Input: part model. Units: mm. Frame: model coordinates. A direction names the side the tool comes from. Round coordinates to 2 decimals unless told otherwise and drop trailing zeros. Loops run counter-clockwise (first coordinate to the right, second up) from the corner with the lowest first, then second, coordinate; pieces in that order, holes last. Notation, with made-up numbers: (-25.75, 66) -> (3.25, 66) arc R22 cw to (3.25, 94) -> close; hole circle Ø6 at (-9.5, 81.5). An arc over 180 degrees is marked (long way). One line per question, with ' | ' between items. Start each with the question number.
Q1. Material intervals for L1, parallel to X at y = 36, z = 0; L2, parallel to Z at x = 0, y = 36; L3, parallel to Y at x = 17.5, z = 17, sorted ascending.
Q2. Cut plane A-A on z = 0. Return loops of the section in (x, y).
Q3. Cut plane B-B on y = 28.5. Return loops of the section in (x, z).
Q4. Cut plane C-C on y = 14. Return loops of the section in (x, z), and give its area (3 significant figures).
Q5. Contact query for flat-ended pins moving along their axis: P1, Ø12, axis at y = 23, z = -3, coming from the +X side; P2, Ø23, axis at x = 0, z = 0, coming from the -Y side; P3, Ø10, axis at x = 15, y = 24, coming from the +Z side; P4, Ø8, axis at x = -14, z = 2.5, coming from the +Y side. Output: stop coordinate, or through.
Q6. Access query for faces 1 (the face through (10, 35, -8)), 2 (the face through (-9.76, 35.99, -2.17)). Directions: +Z, -Z, +X, -X, +Y, -Y. A direction counts if a zero-diameter tool reaches every point of the face in a straight line with its end or side. Return the directions, or none.
Q7. Mould query, pull axis X, two halves, no side actions, for faces 3 (the face through (17, 18, -37)), 4 (the face through (-8.696, 37.313, 5.544)), 5 (the face through (38.738, 38.042, 9.967)), 6 (the face through (-45.84, 2.54, -1.01)). Classes: pulls with the +X half, pulls with the -X half, needs draft (parallel to the pull), parting line crosses it, or undercut.
from build123d import *
from OCP.BRepFilletAPI import BRepFilletAPI_MakeChamfer

# Parameters (mm, degrees)
REVOLVE1_ANGLE          = 180
BOSS_EXTRUDE1_DEPTH     = 60
CUT_EXTRUDE2_DEPTH      = 87.407305825
CUT_EXTRUDE2_DEPTH_BACK = 87.407305825
SKETCH8_R               = 10
BOSS_EXTRUDE2_DEPTH     = 7
CHAMFER1_SIZE           = 5
CHAMFER1_SIZE2          = 6.012778745
CHAMFER2_SIZE           = 1
CHAMFER2_SIZE2          = 0.800998829
CHAMFER2_SIZE2_2        = 1.505173624
CHAMFER2_SIZE2_3        = 0.802603699
CHAMFER2_SIZE2_4        = 1.49466769


with BuildPart() as part:
    # Sketch2 → Revolve1 (revolve)
    with BuildSketch(Plane(origin=(0, 0, 0), x_dir=(0, 0, -1), z_dir=(1, 0, 0))):
        Polygon((37, 0), (45.85, 0), (45.85, 5), (40, 42), (0, 42), (0, 35), (37, 35), align=None)
    revolve(axis=Axis((0, 0, 0), (0, 1, 0)), revolution_arc=REVOLVE1_ANGLE)

    # Sketch7 → Boss-Extrude1 (add)
    with BuildSketch(Plane(origin=(0, 0, 0), x_dir=(0, 0, -1), z_dir=(1, 0, 0))):
        Polygon((-37, 0), (-37, 35), (37, 35), (37, 0), (45.85, 0), (45.85, 5), (40, 42), (-40, 42), (-45.85, 5), (-45.85, 0), align=None)
    extrude(amount=BOSS_EXTRUDE1_DEPTH)

    # Sketch8 → Cut-Extrude2 (cut, two sides: drawn at the far end of the back side and taken through both)
    with BuildSketch(Plane(origin=(0, 0, 0), x_dir=(1, 0, 0), z_dir=(0, 1, 0)).offset(-CUT_EXTRUDE2_DEPTH_BACK)):
        with Locations(Location((0, 0, 0), (0, 0, 270))):
            Circle(SKETCH8_R)
        Polygon((10, -45.85), (38, 45.85), (138, 45.85), (138, -45.85), align=None)
    extrude(amount=CUT_EXTRUDE2_DEPTH + CUT_EXTRUDE2_DEPTH_BACK, mode=Mode.SUBTRACT)

    # Sketch9 → Boss-Extrude2 (add)
    with BuildSketch(Plane(origin=(0, 42, 0), x_dir=(1, 0, 0), z_dir=(0, 1, 0))):
        with BuildLine():
            Line((31.519782555, 24.627287867), (0, -40))
            ThreePointArc((0, -40), (35.951992397, -17.534373175), (31.519782555, 24.627287867))
        make_face()
    extrude(amount=-BOSS_EXTRUDE2_DEPTH)

    # Chamfer1: one chamfer whose edges measure the first distance from different faces: ONE call of the kernel's chamfer builder (chamfer() names one face for all edges)
    chamfer1_edges_1 = [part.edges().sort_by_distance(p)[0] for p in [
        (-40, 42, 0),
        (5.893129771, 42, 40),
        (18.106870229, 42, -40),
    ]]
    chamfer1_side_1 = [part.faces().sort_by_distance(p)[0] for p in [
        (18.106870229, 42, -38.86862915),
    ]]
    chamfer1_edges_2 = [part.edges().sort_by_distance(p)[0] for p in [
        (0, 42, -10),
        (33.866761506, 42, -32.313643934),
    ]]
    chamfer1 = BRepFilletAPI_MakeChamfer(part.part.solid().wrapped)
    for e in chamfer1_edges_1:
        chamfer1.Add(CHAMFER1_SIZE, CHAMFER1_SIZE2, e.wrapped, chamfer1_side_1[0].wrapped)  # the first distance lies on this face
    for e in chamfer1_edges_2:
        chamfer1.Add(CHAMFER1_SIZE, e.wrapped)
    add(Compound.cast(chamfer1.Shape()), mode=Mode.REPLACE)

    # Chamfer2: one chamfer whose edges measure the first distance from different faces: ONE call of the kernel's chamfer builder (chamfer() names one face for all edges)
    chamfer2_edges_1 = [part.edges().sort_by_distance(p)[0] for p in [
        (39.67158228, 42, 5.115228187),
    ]]
    chamfer2_edges_2 = [part.edges().sort_by_distance(p)[0] for p in [
        (12.702290076, 17.5, 37),
    ]]
    chamfer2_side_2 = [part.faces().sort_by_distance(p)[0] for p in [
        (11.622460622, 15.898187568, 40.536441463),
    ]]
    chamfer2_edges_3 = [part.edges().sort_by_distance(p)[0] for p in [
        (35.297709924, 17.5, -37),
    ]]
    chamfer2_side_3 = [part.faces().sort_by_distance(p)[0] for p in [
        (36.103314257, 17.732760886, -39.638354191),
    ]]
    chamfer2_edges_4 = [part.edges().sort_by_distance(p)[0] for p in [
        (37.250229743, 20.530497592, -43.394502408),
    ]]
    chamfer2_side_4 = [part.faces().sort_by_distance(p)[0] for p in [
        (36.103314257, 17.732760886, -39.638354191),
    ]]
    chamfer2_edges_5 = [part.edges().sort_by_distance(p)[0] for p in [
        (10.749770257, 20.530497592, 43.394502408),
    ]]
    chamfer2_side_5 = [part.faces().sort_by_distance(p)[0] for p in [
        (11.622460622, 15.898187568, 40.536441463),
    ]]
    chamfer2 = BRepFilletAPI_MakeChamfer(part.part.solid().wrapped)
    for e in chamfer2_edges_1:
        chamfer2.Add(CHAMFER2_SIZE, e.wrapped)
    for e in chamfer2_edges_2:
        chamfer2.Add(CHAMFER2_SIZE, CHAMFER2_SIZE2, e.wrapped, chamfer2_side_2[0].wrapped)  # the first distance lies on this face
    for e in chamfer2_edges_3:
        chamfer2.Add(CHAMFER2_SIZE, CHAMFER2_SIZE2_2, e.wrapped, chamfer2_side_3[0].wrapped)  # the first distance lies on this face
    for e in chamfer2_edges_4:
        chamfer2.Add(CHAMFER2_SIZE, CHAMFER2_SIZE2_3, e.wrapped, chamfer2_side_4[0].wrapped)  # the first distance lies on this face
    for e in chamfer2_edges_5:
        chamfer2.Add(CHAMFER2_SIZE, CHAMFER2_SIZE2_4, e.wrapped, chamfer2_side_5[0].wrapped)  # the first distance lies on this face
    add(Compound.cast(chamfer2.Shape()), mode=Mode.REPLACE)


solid = part.part
Results:
1) L1: -40.95 to -10, 10 to 40 | L2: -40.95 to -10, 10 to 40.95 | L3: 35 to 42
2) outline: (-45.85, 0) -> (-37, 0) -> (-37, 35) -> (-10, 35) -> (-10, 37) -> (-15, 42) -> (-35, 42) -> (-40.94, 36.06) -> (-45.85, 5) -> close; (10, 35) -> (40, 35) -> (40, 41) -> (39, 42) -> (15, 42) -> (10, 37) -> close
3) outline: (0, -42.13) -> (36.06, -42.13) -> (36.57, -41.17) -> (35.59, -37.96) -> (33.79, -37) -> (0, -37) arc R37 cw to (0, 37) -> (11.9, 37) -> (12.41, 37.96) -> (11.43, 41.17) -> (9.64, 42.13) -> (0, 42.13) arc R42.13 ccw to start
4) outline: (0, -44.43) -> (36.76, -44.43) -> (37.27, -43.46) -> (35.59, -37.96) -> (33.79, -37) -> (0, -37) arc R37 cw to (0, 37) -> (11.9, 37) -> (12.41, 37.96) -> (10.73, 43.46) -> (8.94, 44.43) -> (0, 44.43) arc R44.43 ccw to start | area: 1,300 mm^2
5) P1: x = -35.89 | P2: y = 35 | P3: z = 42.61 | P4: y = 42
6) face 1: +X, -Y | face 2: +Y, -Y
7) face 3: needs draft | face 4: undercut | face 5: pulls with the +X half | face 6: pulls with the -X half
